Can you work these out from the model? Positions are in its coordinate system, mm. Face numbers are marked on the shaded views. A direction names the side the tool comes from. Give positions to 0.01 mm unless a question says otherwise; leave off trailing zeros. Write each loop counter-clockwise with the first axis right and the second up, starting at its lowest first coordinate (ties: lowest second). Pieces come first, ordered by that corner, then holes.
1. Suppose I cut it at C-C (z = 1.75). Please give me the cut outline in (x, y).
2. On a 3-axis mill with a long thin cutter (end or side, diameter ignored), from which of +Z, -Z, +X, -X, +Y, -Y can I reach the whole of each face in a straight line? I mean the marked faces 4 and 5. Say none if no direction works.
3. If I drill on probe 1 along X at (y, z) = (-1, 7); probe 2 along Y at (x, z) = (-1, 7); probe 3 along X at (y, z) = (2.5, 7), over which ranges is the centre line in solid material (lowest first)?
4. Thinking about a two-plate mould opening in X: for the marked faces 1, 2 and 3, which applies, pulls with the +X half, pulls with the -X half, needs draft (parallel to the pull), parting line crosses it, or undercut?
5. I'm going to push flat-ended pins straight in: pin 1 (8 mm diameter, centred on x = 19, z = 5.5, fed in from -Y); pin 2 (2 mm diameter, centred on x = -15.5, z = 3, fed in from -Y); pin 3 (5 mm diameter, centred on x = 5, y = -15, fed in from +Z); pin 4 (8 mm diameter, centred on x = 12.5, y = -18.5, fed in from -Z). Where does each tip first touch, or does it pass through?
6. Suppose I cut it at A-A (z = 10). Give the number of separate pieces and of enclosed holes in the cut face, and give its area (3 significant figures).
```python
from build123d import *

# Parameters (mm, degrees)
F0_R      = 25
F1_DEPTH  = 15
F2_R      = 3
F5_R      = 21.5
F6_DEPTH  = 11
F8_DEPTH  = 10.8
F9_R      = 26.2697313625
F9_R_2    = 23
F10_DEPTH = 5.7
F11_W     = 62.843285501
F11_H     = 17.6012022421
F12_DEPTH = 30


with BuildPart() as f1:
    # F0 (on Top) → F1 (new body)
    with BuildSketch(Plane.XY):
        Circle(F0_R)
    extrude(amount=F1_DEPTH)

    # F2
    f2_edges = [f1.edges().sort_by_distance(p)[0] for p in [
        (-25, 0, 0),
    ]]
    fillet(f2_edges, radius=F2_R)

    # F3 (on Front) → F4 (revolve, cut)
    with BuildSketch(Plane.XZ):
        with BuildLine():
            Line((27.423677966, 5.2825664575), (25, 14.9365440011))
            add(Edge.make_bspline(
                [(25, 14.9365440011), (24.5482466845, 13.0284596048), (23.6395446157, 9.1903466819), (24.5447896478, 5.2825664575), (25, 3.3175051212)],
                knots=[0, 0, 0, 0, 0.4971412865, 1, 1, 1, 1], degree=3))
            Line((25, 3.3175051212), (27.423677966, 5.2825664575))
        make_face()
    revolve(axis=Axis((0, 0, 20.2008970082), (0, 0, -1)), mode=Mode.SUBTRACT)

    # F5 (on face) → F6 (cut)
    with BuildSketch(Plane.XY.offset(15)):
        Circle(F5_R)
    extrude(amount=-F6_DEPTH, mode=Mode.SUBTRACT)

    # F7 (on face) → F8 (join)
    with BuildSketch(Plane.XY.offset(4)):
        with BuildLine():
            Line((-3.5030060365, 4.8188975732), (-3.5, 4.8173367216))
            Line((-3.5, 4.8173367216), (-3.4936811056, 4.8173367216))
            ThreePointArc((-3.4936811056, 4.8173367216), (-3.4985674675, 4.8197108468), (-3.5034522162, 4.8220882896))
            ThreePointArc((-3.5034522162, 4.8220882896), (-3.5032289657, 4.8204929538), (-3.5030060365, 4.8188975732))
        make_face()
        with BuildLine():
            Line((-3.5019526458, 4.8113270959), (-3.5, 4.8173367216))
            Line((-3.5, 4.8173367216), (-3.5030060365, 4.8188975732))
            ThreePointArc((-3.5030060365, 4.8188975732), (-3.502478437, 4.8151124604), (-3.5019526458, 4.8113270959))
        make_face()
        with BuildLine():
            Line((-3.4936811056, 4.8173367216), (-3.5, 4.8173367216))
            Line((-3.5, 4.8173367216), (-3.5019526458, 4.8113270959))
            ThreePointArc((-3.5019526458, 4.8113270959), (-3.8176882042, 1.2404420916), (-5.6611663149, -1.8340492667))
            Line((-5.6611663149, -1.8340492667), (-5.6631189606, -1.8400588924))
            Line((-5.6631189606, -1.8400588924), (-5.6580068676, -1.8437730454))
            ThreePointArc((-5.6580068676, -1.8437730454), (-2.3594610686, -3.2475195569), (-0.005112093, -5.9508415055))
            Line((-0.005112093, -5.9508415055), (0, -5.9545556585))
            Line((0, -5.9545556585), (0.005112093, -5.9508415055))
            ThreePointArc((0.005112093, -5.9508415055), (0.0154537536, -5.9315416501), (0.025848199, -5.912270172))
            Line((0.025848199, -5.912270172), (0.0131157498, -2.9999713294))
            ThreePointArc((0.0131157498, -2.9999713294), (-2.9999928323, -0.0065578905), (0, 3))
            Line((0, 3), (0, 4.0141549306))
            ThreePointArc((0, 4.0141549306), (-1.7924082025, 4.2175356096), (-3.4936811056, 4.8173367216))
        make_face()
        Polygon((-3, 12.0141549306), (0, 10.6355519965), (0, 12.0141549306), (3, 12.0141549306), (0, 13.3927578647), align=None)
        Polygon((0, 12.0141549306), (0, 10.6355519965), (3, 12.0141549306), align=None)
        Polygon((3.9177863585, -21.4830770759), (0.0836216544, -19.1268185495), (0.0939962066, -21.4997945272), align=None)
        Polygon((0.0939962066, -21.4997945272), (0.0836216544, -19.1268185495), (-3.7297939454, -21.5165119786), align=None)
        with BuildLine():
            Line((-3.6865685479, 4.9142103997), (-3.5030060365, 4.8188975732))
            ThreePointArc((-3.5030060365, 4.8188975732), (-3.5032289657, 4.8204929538), (-3.5034522162, 4.8220882896))
            ThreePointArc((-3.5034522162, 4.8220882896), (-3.5953054485, 4.8675628244), (-3.6865685479, 4.9142103997))
        make_face()
        with BuildLine():
            ThreePointArc((3.5034522162, 4.8220882896), (1.7977022656, 4.218754584), (0, 4.0141549306))
            Line((0, 4.0141549306), (0, 3))
            ThreePointArc((0, 3), (2.1213203436, 2.1213203436), (3, 0))
            ThreePointArc((3, 0), (2.1259524041, -2.1166781464), (0.0131157498, -2.9999713294))
            Line((0.0131157498, -2.9999713294), (0.025848199, -5.912270172))
            ThreePointArc((0.025848199, -5.912270172), (2.3771928926, -3.2346736711), (5.6580068676, -1.8437730454))
            Line((5.6580068676, -1.8437730454), (5.6631189606, -1.8400588924))
            Line((5.6631189606, -1.8400588924), (5.6611663149, -1.8340492667))
            ThreePointArc((5.6611663149, -1.8340492667), (3.8176882042, 1.2404420916), (3.5019526458, 4.8113270959))
            Line((3.5019526458, 4.8113270959), (3.5, 4.8173367216))
            Line((3.5, 4.8173367216), (3.5030060365, 4.8188975732))
            ThreePointArc((3.5030060365, 4.8188975732), (3.5032289657, 4.8204929538), (3.5034522162, 4.8220882896))
        make_face()
        with BuildLine():
            Line((-5.6631189606, -1.8400588924), (-5.6611663149, -1.8340492667))
            ThreePointArc((-5.6611663149, -1.8340492667), (-5.6649342109, -1.8379628281), (-5.6687047637, -1.8418738299))
            ThreePointArc((-5.6687047637, -1.8418738299), (-5.6633554933, -1.8428216215), (-5.6580068676, -1.8437730454))
            Line((-5.6580068676, -1.8437730454), (-5.6631189606, -1.8400588924))
        make_face()
        with BuildLine():
            ThreePointArc((3.6865685479, 4.9142103997), (3.5953054485, 4.8675628244), (3.5034522162, 4.8220882896))
            ThreePointArc((3.5034522162, 4.8220882896), (3.5032289657, 4.8204929538), (3.5030060365, 4.8188975732))
            Line((3.5030060365, 4.8188975732), (3.6865685479, 4.9142103997))
        make_face()
        with BuildLine():
            ThreePointArc((3.5019526458, 4.8113270959), (3.502478437, 4.8151124604), (3.5030060365, 4.8188975732))
            Line((3.5030060365, 4.8188975732), (3.5, 4.8173367216))
            Line((3.5, 4.8173367216), (3.5019526458, 4.8113270959))
        make_face()
        with BuildLine():
            Line((0.0259506395, -5.9357014153), (0.025848199, -5.912270172))
            ThreePointArc((0.025848199, -5.912270172), (0.0154537536, -5.9315416501), (0.005112093, -5.9508415055))
            Line((0.005112093, -5.9508415055), (0.0259506395, -5.9357014153))
        make_face()
        with BuildLine():
            Line((0, -5.9545556585), (-0.005112093, -5.9508415055))
            ThreePointArc((-0.005112093, -5.9508415055), (-0.0025544188, -5.9556343446), (0, -5.9604289194))
            ThreePointArc((0, -5.9604289194), (0.0025544188, -5.9556343446), (0.005112093, -5.9508415055))
            Line((0.005112093, -5.9508415055), (0, -5.9545556585))
        make_face()
        with BuildLine():
            ThreePointArc((5.6687047637, -1.8418738299), (5.6649342109, -1.8379628281), (5.6611663149, -1.8340492667))
            Line((5.6611663149, -1.8340492667), (5.6631189606, -1.8400588924))
            Line((5.6631189606, -1.8400588924), (5.6580068676, -1.8437730454))
            ThreePointArc((5.6580068676, -1.8437730454), (5.6633554933, -1.8428216215), (5.6687047637, -1.8418738299))
        make_face()
        with BuildLine():
            Line((0.0259506395, -5.9357014153), (0.005112093, -5.9508415055))
            ThreePointArc((0.005112093, -5.9508415055), (0.0025544188, -5.9556343446), (0, -5.9604289194))
            ThreePointArc((0, -5.9604289194), (0.0131819815, -5.9852967616), (0.0262763915, -6.0102108267))
            Line((0.0262763915, -6.0102108267), (0.0259506395, -5.9357014153))
        make_face()
        Polygon((-12.7372696383, 4.1385897817), (-12.3531913176, 0.8594084977), (-10.1150110307, 3.2865663115), (-10.4990893514, 6.5657475955), align=None)
        Polygon((-7.8720655604, -10.8349687141), (-4.6346921038, -11.4830112688), (-6.2514206135, -8.6043423098), (-9.4887940701, -7.956299755), align=None)
        Polygon((7.8720655604, -10.8349687141), (9.4887940701, -7.956299755), (6.2514206135, -8.6043423098), (4.6346921038, -11.4830112688), align=None)
        Polygon((12.7372696383, 4.1385897817), (10.4990893514, 6.5657475955), (10.1150110307, 3.2865663115), (12.3531913176, 0.8594084977), align=None)
        Polygon((16.8678219042, -13.3314134363), (19.2388458386, -10.3314307527), (15.0060861502, -11.8599982656), (14.4967979698, -16.3313961198), align=None)
        Polygon((20.9398336671, 4.8757938835), (20.0726620013, 8.5999936501), (18.6286617065, 4.3376426122), (21.8070053329, 1.1515941169), align=None)
        Polygon((9.2437235839, 19.4114289609), (5.7913542693, 21.0554474264), (8.2234750424, 17.2689501312), (12.6960928985, 17.7674104954), align=None)
        Polygon((-9.4130988956, 19.3298621098), (-12.8509613495, 17.6557198378), (-8.374156057, 17.1963859791), (-5.9752364416, 21.0040043817), align=None)
        Polygon((-20.9816659144, 4.6925148326), (-21.8162409604, 0.9608751003), (-18.6658768438, 4.1745924423), (-20.1470908685, 8.424154565), align=None)
        Polygon((-16.7506105518, -13.4783918233), (-14.3534461578, -16.457528186), (-14.9018116527, -11.9907543496), (-19.1477749457, -10.4992554606), align=None)
    extrude(amount=F8_DEPTH)

    # F9 (on face) → F10 (cut)
    with BuildSketch(Plane.XY.offset(15)):
        Circle(F9_R)
        Circle(F9_R_2, mode=Mode.SUBTRACT)
    extrude(amount=-F10_DEPTH, mode=Mode.SUBTRACT)

    # F11 (on Right) → F12 (cut, symmetric)
    with BuildSketch(Plane.YZ):
        with Locations((-2.5946311653, 23.1964425184)):
            Rectangle(F11_W, F11_H)
    extrude(amount=F12_DEPTH, both=True, mode=Mode.SUBTRACT)


solid = f1.part
```
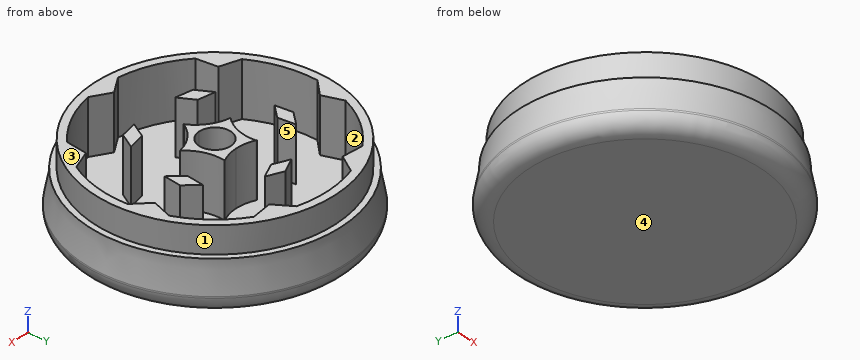
Checks:
1. outline: circle Ø49.45 at (0, 0)
2. face 4: -Z, +X, -X, +Y, -Y
2. face 5: +Z
3. probe 1: x = -24.24 to -21.48, -4.96 to -2.83, 2.83 to 4.96, 21.48 to 24.24
3. probe 2: y = -24.24 to -19.81, -4.5 to -2.83, 2.83 to 4.08, 11.1 to 12.93, 21.48 to 24.24
3. probe 3: x = -24.13 to -20.31, -12.55 to -10.84, -3.52 to -1.66, 1.66 to 3.52, 10.84 to 12.55, 20.46 to 24.13
4. face 1: parting line crosses it
4. face 2: undercut
4. face 3: needs draft
5. pin 1: stops at y = -19.58
5. pin 2: stops at y = -20.37
5. pin 3: stops at z = 4
5. pin 4: stops at z = 0
6. separate pieces: 7
6. enclosed holes: 2
6. area: 347 mm2
